Geometry: see drawing. Coordinates: mm, zero at the bounding-box minimum. A direction names the side the tool comes from. Give positions to 0.01 mm unless a question says otherwise; leave off trailing zeros. Write each loop counter-clockwise with the first axis right and the second up, starting at its lowest first coordinate (ties: lowest second). Pieces come first, ordered by that corner, then holes. Notation, with made-up numbers: M -39,-29 L -22,-29 A22 ccw -22,-23 Z; hole C 59.25,57.5 d10. An arc over 180 degrees is marked long. Use a Markdown table: item, result. Add a question column.
1) Section A-A on y = 28. Return the cut outline in (x, z).
2) Set-up query: the marked faces 4, 5, 6 and 7. Return all of +Z, -Z, +X, -X, +Y, -Y with unobstructed straight access to the full face (end or side cutting, diameter ignored); none if empty.
3) Section B-B on z = 47.5. Return the cut outline in (x, y).
4) Draft query along X for the marked faces 1, 2 and 3. Return one class per face: +X half, -X half, draft (parallel to the pull), parting line (faces both ways), or undercut.
5) Pin query (flat end, axial travel): pin 1 (8 mm diameter, centred on x = 61, z = 33, fed in from -Y); pin 2 (6 mm diameter, centred on x = 25, z = 26.5, fed in from -Y); pin 3 (10 mm diameter, centred on x = 41.5, z = 24, fed in from -Y). Return the tip coordinate at first contact, or that it passes through.
6) Line query: line 1 (X direction, y = 30, z = 39.5); line 2 (X direction, y = 23.5, z = 24.5); line 3 (Y direction, x = 7, z = 21). Output: solid intervals per line, ascending.
7) Section C-C on z = 31. Return the cut outline in (x, y), then the cut area to 3 significant figures.
8) Section D-D on y = 43.5. Return the cut outline in (x, z).
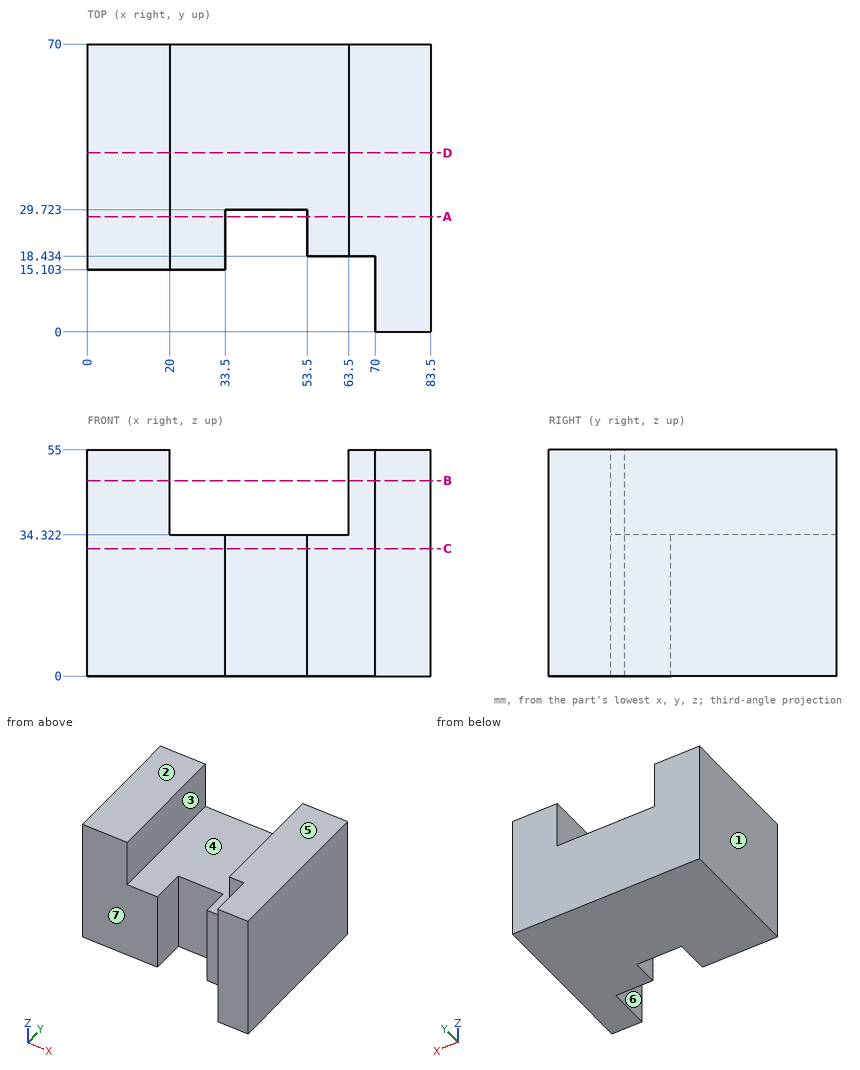
Found:
| question | item | result |
|---|---|---|
| 1 | outline | M 0,0 L 33.5,0 L 33.5,34.32 L 20,34.32 L 20,55 L 0,55 Z; M 53.5,0 L 83.5,0 L 83.5,55 L 63.5,55 L 63.5,34.32 L 53.5,34.32 Z |
| 2 | face 4 | +Z, +Y, -Y |
| 2 | face 5 | +Z, +X, -X, +Y, -Y |
| 2 | face 6 | +Z, -Z, -Y |
| 2 | face 7 | +Z, -Z, -X, -Y |
| 3 | outline | M 0,15.1 L 20,15.1 L 20,70 L 0,70 Z; M 63.5,18.43 L 70,18.43 L 70,0 L 83.5,0 L 83.5,70 L 63.5,70 Z |
| 4 | face 1 | -X half |
| 4 | face 2 | draft |
| 4 | face 3 | undercut |
| 5 | pin 1 | y = 18.43 |
| 5 | pin 2 | y = 15.1 |
| 5 | pin 3 | y = 29.72 |
| 6 | line 1 | 0 to 20, 63.5 to 83.5 |
| 6 | line 2 | 0 to 33.5, 53.5 to 83.5 |
| 6 | line 3 | 15.1 to 70 |
| 7 | outline | M 0,15.1 L 33.5,15.1 L 33.5,29.72 L 53.5,29.72 L 53.5,18.43 L 70,18.43 L 70,0 L 83.5,0 L 83.5,70 L 0,70 Z |
| 7 | area | 4,440 mm² |
| 8 | outline | M 0,0 L 83.5,0 L 83.5,55 L 63.5,55 L 63.5,34.32 L 20,34.32 L 20,55 L 0,55 Z |
